Here's how the part is built. I have some questions about the finished solid (model axes, mm). Face numbers are marked on the shaded views. A direction names the side the tool comes from. Round coordinates to 2 decimals unless told otherwise and drop trailing zeros. Write each loop counter-clockwise with the first axis right and the second up, starting at its lowest first coordinate (ties: lowest second). Pieces come first, ordered by that corner, then holes. Notation, with made-up numbers: (59.25, 21.5) - (83.25, 21.5) arc R14 ccw to (83.25, 33.5) - close; hole circle Ø8 at (83.5, 51.5). An arc over 180 degrees is marked (long way). Write item = value, one per line. Start each with the question number.
Item 1: If we section it at A-A (y = -41.25): Please give me the cut outline in (x, z), and give its area (4 significant figures).
Item 2: If we section it at D-D (x = -30): Please give me the cut outline in (y, z), and give its area (3 significant figures).
Item 3: If we section it at C-C (z = 10): Please give me the cut outline in (x, y), and give its area (3 significant figures).
Item 4: If I drill on line 1 along Y through (x, z) = (-64, 1.7); line 2 along Y through (x, z) = (15, 1); line 3 along X through (y, z) = (-84.5, 32), over which ranges is the centre line in solid material (lowest first)? Write a range as [from, to].
Item 5: If we section it at B-B (x = 15): Please give me the cut outline in (y, z).
Item 6: For P1, Ø13.5, axis at y = -66.5, z = 15, coming from the +X side; P2, Ø17.5, axis at y = -64, z = 25, coming from the -X side; P3, Ø13.5, axis at y = -46.5, z = 33.5, coming from the -X side; P4, Ø8, axis at x = -54.5, z = 8, coming from the +Y side, each with a flat end and sliding along its axis, tell me the tip position at first contact or that it passes through.
Item 7: Thinking about a two-plate mould opening in Z: for the marked faces 4, 5 and 6, which applies, pulls with the +Z half, pulls with the -Z half, needs draft (parallel to the pull), parting line crosses it, or undercut?
Item 8: Which directions (+Z, -Z, +X, -X, +Y, -Y) give clear straight access to the entire face, cutting with the end or side of a thin tool? Please do the marked faces 1, 2 and 3.
```python
from build123d import *

# Parameters (mm, degrees)
SKETCH2_R             = 2.75
BOSS_EXTRUDE1_DEPTH   = 5
BOSS_EXTRUDE1_2_DEPTH = 5
BOSS_EXTRUDE3_DEPTH   = 2.5
BOSS_EXTRUDE4_DEPTH   = 2.5
BOSS_EXTRUDE5_DEPTH   = 5
BOSS_EXTRUDE6_DEPTH   = 5
FILLET1_R             = 5
FILLET2_R             = 5
FILLET3_R             = 5
FILLET4_R             = 5
SKETCH7_R             = 5
BOSS_EXTRUDE7_DEPTH   = 49
BOSS_EXTRUDE8_START   = 49
SKETCH8_R             = 5
BOSS_EXTRUDE8_DEPTH   = 49


with BuildPart() as part:
    # Sketch2 → Boss-Extrude1 (new body)
    with BuildSketch(Plane.XY):
        Polygon((-10, -75), (-10, -115), (20, -115), (20, -30), (5, -30), (5, -75), align=None)
        with Locations((15, -35.919713403)):
            Circle(SKETCH2_R, mode=Mode.SUBTRACT)
        with Locations((15, -65)):
            Circle(SKETCH2_R, mode=Mode.SUBTRACT)
    extrude(amount=BOSS_EXTRUDE1_DEPTH)

    # Sketch4 → Boss-Extrude4 (add)
    with BuildSketch(Plane.ZY.offset(-5)):
        Polygon((0, -30), (0, -75), (5, -75), (5, -85), (53.715728753, -85), (18.715728753, -50), (5, -50), (5, -30), align=None)
    extrude(amount=-BOSS_EXTRUDE4_DEPTH)

    # Sketch6 → Boss-Extrude6 (add)
    with BuildSketch(Plane.ZY.offset(-5)):
        Polygon((0, -30), (0, -75), (5, -75), (5, -85), (53.715728753, -85), (18.715728753, -50), (5, -50), (5, -30), align=None)
    extrude(amount=BOSS_EXTRUDE6_DEPTH)

    # Fillet1
    fillet1_edges = [part.edges().sort_by_distance(p)[0] for p in [
        (3.75, -85, 53.715728753),
    ]]
    fillet(fillet1_edges, radius=FILLET1_R)

    # Fillet4
    fillet4_edges = [part.edges().sort_by_distance(p)[0] for p in [
        (3.75, -50, 18.715728753),
    ]]
    fillet(fillet4_edges, radius=FILLET4_R)



with BuildPart() as body_2:
    # Sketch2 → Boss-Extrude1 2 (new body)
    with BuildSketch(Plane.XY):
        Polygon((-74, -30), (-74, -115), (-44, -115), (-44, -75), (-54, -75), (-54, -30), align=None)
        with Locations((-64, -65)):
            Circle(SKETCH2_R, mode=Mode.SUBTRACT)
        with Locations((-64, -41.25)):
            Circle(SKETCH2_R, mode=Mode.SUBTRACT)
    extrude(amount=BOSS_EXTRUDE1_2_DEPTH)

    # Sketch3 → Boss-Extrude3 (add)
    with BuildSketch(Plane(origin=(-54, 0, 0), x_dir=(0, 0, -1), z_dir=(1, 0, 0))):
        Polygon((-5, -75), (-5, -50), (-18.715728753, -50), (-53.715728753, -85), (-5, -85), align=None)
    extrude(amount=-BOSS_EXTRUDE3_DEPTH)

    # Sketch5 → Boss-Extrude5 (add)
    with BuildSketch(Plane(origin=(-54, 0, 0), x_dir=(0, 0, -1), z_dir=(1, 0, 0))):
        Polygon((0, -75), (0, -30), (-5, -30), (-5, -50), (-18.715728753, -50), (-53.715728753, -85), (-5, -85), (-5, -75), align=None)
    extrude(amount=BOSS_EXTRUDE5_DEPTH)

    # Fillet2
    fillet2_edges = [body_2.edges().sort_by_distance(p)[0] for p in [
        (-52.75, -85, 53.715728753),
    ]]
    fillet(fillet2_edges, radius=FILLET2_R)

    # Fillet3
    fillet3_edges = [body_2.edges().sort_by_distance(p)[0] for p in [
        (-52.75, -50, 18.715728753),
    ]]
    fillet(fillet3_edges, radius=FILLET3_R)


with BuildPart() as part_1:
    add(part.part)

    add(body_2.part)  # Boss-Extrude7 merges body 2
    # Sketch7 → Boss-Extrude7 (add)
    with BuildSketch(Plane(origin=(-49, 0, 0), x_dir=(0, 0, -1), z_dir=(1, 0, 0))):
        with Locations(Location((-41.644660941, -80, 0), (0, 0, 135))):
            Circle(SKETCH7_R)
    extrude(amount=BOSS_EXTRUDE7_DEPTH)

    # Sketch8 → Boss-Extrude8 (add)
    with BuildSketch(Plane(origin=(-49, 0, 0), x_dir=(0, 0, -1), z_dir=(1, 0, 0)).offset(BOSS_EXTRUDE8_START)):
        with Locations(Location((-16.644660941, -55, 0), (0, 0, 90))):
            Circle(SKETCH8_R)
    extrude(amount=-BOSS_EXTRUDE8_DEPTH)


solid = part_1.part
```
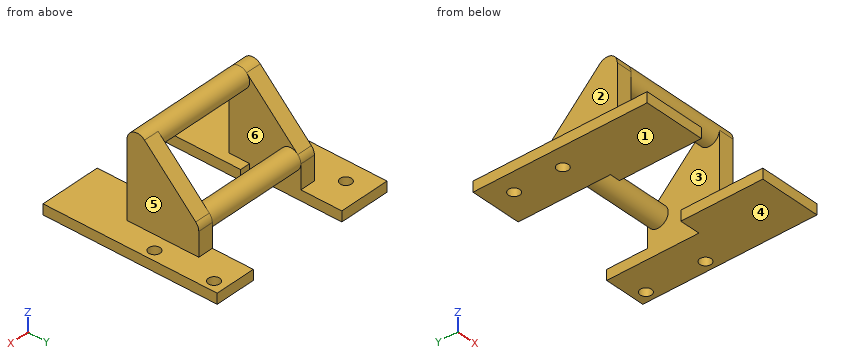
Reply:
q1.outline = (-74, 0) - (-66.75, 0) - (-66.75, 5) - (-74, 5) - close; (-61.25, 0) - (-49, 0) - (-49, 5) - (-61.25, 5) - close; (0, 0) - (20, 0) - (20, 5) - (0, 5) - close
q1.area = 197.5 mm2
q2.outline = circle Ø10 at (-80, 41.64); circle Ø10 at (-55, 16.64)
q2.area = 157 mm2
q3.outline = (-56.5, -85) - (-49, -85) - (-49, -50) - (-56.5, -50) - close; (0, -85) - (7.5, -85) - (7.5, -50) - (0, -50) - close
q3.area = 525 mm2
q4.line_1 = [-115, -67.75], [-62.25, -44], [-38.5, -30]
q4.line_2 = [-115, -67.75], [-62.25, -38.67], [-33.17, -30]
q4.line_3 = [-56.5, -49], [0, 7.5]
q5.outline = (-115, 0) - (-67.75, 0) - (-67.75, 5) - (-115, 5) - close; (-62.25, 0) - (-38.67, 0) - (-38.67, 5) - (-62.25, 5) - close; (-33.17, 0) - (-30, 0) - (-30, 5) - (-33.17, 5) - close
q6.P1 = 7.5
q6.P2 = -56.5
q6.P3 = through
q6.P4 = -30
q7.face_4 = pulls with the -Z half
q7.face_5 = needs draft
q7.face_6 = undercut
q8.face_1 = -Z, +X, -X, +Y, -Y
q8.face_2 = +Z, -X, +Y, -Y
q8.face_3 = none
